```python
from build123d import *

# Parameters (mm, degrees)
F1_DEPTH = 110
F2_R     = 1.75
F3_DEPTH = 8
F4_R     = 2
F5_DEPTH = 10
F6_R     = 5


with BuildPart() as f1:
    # F0 (on Right) → F1 (new body)
    with BuildSketch(Plane.YZ):
        Polygon((60, 5.6479252494), (6.3304924375, 5.6479252494), (24.7478693281, 37.5477577661), (20, 40.2889414007), (0, 5.6479252494), (0, 0), (60, 0), align=None)
    extrude(amount=F1_DEPTH)

    # F2 (on face) → F3 (cut)
    with BuildSketch(Plane(origin=(0, -2.4456233723, 1.4119813123), x_dir=(1, 0, 0), z_dir=(0, -0.8660254038, 0.5))):
        with Locations((11.5, 26.8912467446)):
            Circle(F2_R)
        with Locations((98.5, 26.8912467446)):
            Circle(F2_R)
    extrude(amount=-F3_DEPTH, mode=Mode.SUBTRACT)

    # F4 (on face) → F5 (cut)
    with BuildSketch(Plane.XY.offset(5.6479252494)):
        with Locations((100, 50)):
            Circle(F4_R)
        with Locations((55, 50.1541644335)):
            Circle(F4_R)
        with Locations((10, 50)):
            Circle(F4_R)
    extrude(amount=-F5_DEPTH, mode=Mode.SUBTRACT)

    # F6
    f6_edges = [f1.edges().sort_by_distance(p)[0] for p in [
        (55, 0, 5.647925),
    ]]
    fillet(f6_edges, radius=F6_R)


solid = f1.part
```
CAD build for the part. Positions are in the model's coordinates, mm. A direction names the side the tool comes from. Round coordinates to 2 decimals unless told otherwise and drop trailing zeros. Write each loop counter-clockwise with the first axis right and the second up, starting at its lowest first coordinate (ties: lowest second). Pieces come first, ordered by that corner, then holes. Notation, with made-up numbers: (79.5, -26) - (118.5, -26) arc R30 ccw to (118.5, 0) - close; hole circle Ø5 at (-23.5, 20). An arc over 180 degrees is marked (long way). Write item = value, one per line. Start each with the question number.
Q1. Band-saw the part on C-C (z = 16). Give the cut face in (x, y).
Q2. Band-saw the part on A-A (x = 55). Give the cut face in (y, z).
Q3. Mould opens along Z. For faces 3 (the cylindrical face through (98.12, 12.49, 21.87)), 4 (the cylindrical face through (55.77, 0.175, 5.62)), 5 (the cylindrical face through (10.923, 48.226, 2.863)), 6 (the flat face through (54.23, 15.41, 21.375)) say: pulls with the +Z half, pulls with the -Z half, needs draft (parallel to the pull), parting line crosses it, or undercut.
Q4. Probe L1, parallel to Y at x = 55, z = 2.45; L2, parallel to Y at x = 10, z = 2.7; L3, parallel to Z at x = 17, y = 36. List the from-to ranges inside material, lowest first. Write a range as from..to.
Q5. Drop flat-ended pins along their axis: pin 1 (10 mm diameter, centred on x = 16.5, z = 25.5, fed in from +Y); pin 2 (6 mm diameter, centred on x = 74.5, y = 52.5, fed in from +Z); pin 3 (1 mm diameter, centred on y = 7, z = 22.5, fed in from -X); pin 4 (8 mm diameter, centred on x = 78.5, z = 12, fed in from -Y). Give the stop position or say it passes through.
Q6. Which spindle directions (+Z, -Z, +X, -X, +Y, -Y) get a long thin tool onto all of the face, cutting with end or side? Do faces 1 (the flat face through (54, 34, 5.648)), 2 (the flat face through (0, 23, 5)). Say none if no direction does.
Q7. Band-saw the part on B-B (y = 34). Give the cut face in (x, z), then the cut area to 3 significant figures.
Answers below:
q1.outline = (0, 5.98) - (110, 5.98) - (110, 12.31) - (0, 12.31) - close
q2.outline = (0, 0) - (48.15, 0) - (48.15, 5.65) - (6.33, 5.65) - (24.75, 37.55) - (20, 40.29) - (0.67, 6.81) arc R5 ccw to (0, 4.31) - close; (52.15, 0) - (60, 0) - (60, 5.65) - (52.15, 5.65) - close
q3.face_3 = undercut
q3.face_4 = pulls with the +Z half
q3.face_5 = needs draft
q3.face_6 = undercut
q4.L1 = 0..48.15, 52.15..60
q4.L2 = 0..48, 52..60
q4.L3 = 0..5.65
q5.pin_1 = 20.68
q5.pin_2 = 5.65
q5.pin_3 = through
q5.pin_4 = 1.36
q6.face_1 = +X, -X, +Y
q6.face_2 = +Z, -Z, -X, +Y, -Y
q7.outline = (0, 0) - (110, 0) - (110, 5.65) - (0, 5.65) - close
q7.area = 621 mm2
